Work out the finished part from the listing and answer in its coordinate system (mm). A direction names the side the tool comes from. Round coordinates to 2 decimals unless told otherwise and drop trailing zeros. Order: outer loops, then holes, each group sorted by start corner. A loop starts at its lowest first (then second) coordinate and runs counter-clockwise, first axis right, second up. Notation, with made-up numbers: M 40.5,46 L 92.5,46 A28 ccw 92.5,71 Z; hole C 69.5,66.25 d3. An arc over 180 degrees is marked long. Return JSON: item names as keys, results as strings.
from build123d import *

# Parameters (mm, degrees)
SKETCH1_R             = 14.29385
SKETCH1_R_2           = 11.1125
BOSS_EXTRUDE1_DEPTH   = 6.35
CROQUIS1_R            = 2.38125
CORTAR_EXTRUIR1_DEPTH = 50
CROQUIS2_R            = 5
CORTAR_EXTRUIR2_DEPTH = 3.175
CROQUIS4_R            = 5
CORTAR_EXTRUIR3_DEPTH = 3.175
CROQUIS5_R            = 2.38125
CORTAR_EXTRUIR5_DEPTH = 10
CROQUIS6_R            = 2.38125
CORTAR_EXTRUIR6_DEPTH = 10
CROQUIS7_R            = 5
CORTAR_EXTRUIR7_DEPTH = 3.17
CROQUIS8_R            = 17.5
CORTAR_EXTRUIR8_DEPTH = 10
CROQUIS9_R            = 2.5527
CORTAR_EXTRUIR9_DEPTH = 10


with BuildPart() as part:
    # Sketch1 → Boss-Extrude1 (new body)
    with BuildSketch(Plane.XY):
        with BuildLine():
            Line((0, 70), (310, 45))
            ThreePointArc((310, 45), (355, 0), (310, -45))
            Line((310, -45), (5.171398252, -69.808714643))
            ThreePointArc((5.171398252, -69.808714643), (-69.952162315, -2.587467389), (0, 70))
        make_face()
        Circle(SKETCH1_R, mode=Mode.SUBTRACT)
        with Locations((310, 0)):
            Circle(SKETCH1_R, mode=Mode.SUBTRACT)
        with Locations((162.878542763, 35)):
            Circle(SKETCH1_R_2, mode=Mode.SUBTRACT)
        with BuildLine():
            Line((107.898974887, 49.259511156), (143.314248041, 46.40344074))
            ThreePointArc((143.314248041, 46.40344074), (147.389908855, 43.644764005), (147.127454118, 38.730252238))
            Line((147.127454118, 38.730252238), (129.916226305, 11.754586611))
            ThreePointArc((129.916226305, 11.754586611), (125.651076231, 9.444205574), (121.433006579, 11.839462159))
            Line((121.433006579, 11.839462159), (103.228961238, 41.671198203))
            ThreePointArc((103.228961238, 41.671198203), (103.238833139, 46.896293531), (107.898974887, 49.259511156))
        make_face(mode=Mode.SUBTRACT)
        with BuildLine():
            Line((70.523244027, 6), (102.03004784, 6))
            ThreePointArc((102.03004784, 6), (106.3902351, 8.552804247), (106.298140539, 13.604493178))
            Line((106.298140539, 13.604493178), (96.590354482, 29.513051181))
            ThreePointArc((96.590354482, 29.513051181), (88.437172177, 34.296727565), (79.941746192, 30.151166228))
            Line((79.941746192, 30.151166228), (65.58297828, 10.229432452))
            ThreePointArc((65.58297828, 10.229432452), (67.271539685, 7.201787411), (70.523244027, 6))
        make_face(mode=Mode.SUBTRACT)
        with BuildLine():
            Line((219.623774494, 32.810522613), (206.130928429, 12.417497436))
            ThreePointArc((206.130928429, 12.417497436), (201.919524559, 10.176643248), (197.745901529, 12.48710226))
            Line((197.745901529, 12.48710226), (183.296864227, 35.133505128))
            ThreePointArc((183.296864227, 35.133505128), (183.227765467, 40.400743015), (187.913912204, 42.80669363))
            Line((187.913912204, 42.80669363), (215.855795571, 40.553315939))
            ThreePointArc((215.855795571, 40.553315939), (219.949772588, 37.757395035), (219.623774494, 32.810522613))
        make_face(mode=Mode.SUBTRACT)
        with BuildLine():
            Line((96.590354482, -29.513051181), (106.298140539, -13.604493178))
            ThreePointArc((106.298140539, -13.604493178), (106.3902351, -8.552804247), (102.03004784, -6))
            Line((102.03004784, -6), (70.523244027, -6))
            ThreePointArc((70.523244027, -6), (67.271539685, -7.201787411), (65.58297828, -10.229432452))
            Line((65.58297828, -10.229432452), (79.941746192, -30.151166228))
            ThreePointArc((79.941746192, -30.151166228), (88.437172177, -34.296727565), (96.590354482, -29.513051181))
        make_face(mode=Mode.SUBTRACT)
        with BuildLine():
            Line((187.913912204, -42.80669363), (215.855795571, -40.553315939))
            ThreePointArc((215.855795571, -40.553315939), (219.949772588, -37.757395035), (219.623774494, -32.810522613))
            Line((219.623774494, -32.810522613), (206.130928429, -12.417497436))
            ThreePointArc((206.130928429, -12.417497436), (201.919524559, -10.176643248), (197.745901529, -12.48710226))
            Line((197.745901529, -12.48710226), (183.296864227, -35.133505128))
            ThreePointArc((183.296864227, -35.133505128), (183.227765467, -40.400743015), (187.913912204, -42.80669363))
        make_face(mode=Mode.SUBTRACT)
        with BuildLine():
            Line((121.433006579, -11.839462159), (103.228961238, -41.671198203))
            ThreePointArc((103.228961238, -41.671198203), (103.238833139, -46.896293531), (107.898974887, -49.259511156))
            Line((107.898974887, -49.259511156), (143.314248041, -46.40344074))
            ThreePointArc((143.314248041, -46.40344074), (147.389908855, -43.644764005), (147.127454118, -38.730252238))
            Line((147.127454118, -38.730252238), (129.916226305, -11.754586611))
            ThreePointArc((129.916226305, -11.754586611), (125.651076231, -9.444205574), (121.433006579, -11.839462159))
        make_face(mode=Mode.SUBTRACT)
    extrude(amount=BOSS_EXTRUDE1_DEPTH)

    # Croquis1 → Cortar-Extruir1 (cut)
    with BuildSketch(Plane.XY.offset(6.35)):
        with Locations((98.995555235, -37.090103176)):
            Circle(CROQUIS1_R)
        with Locations((228.877351461, -26.519571404)):
            Circle(CROQUIS1_R)
    extrude(amount=-CORTAR_EXTRUIR1_DEPTH, mode=Mode.SUBTRACT)

    # Croquis2 → Cortar-Extruir2 (cut)
    with BuildSketch(Plane.XY.offset(6.35)):
        with Locations((98.995555235, -37.090103176)):
            Circle(CROQUIS2_R)
        with Locations((228.877351461, -26.519571404)):
            Circle(CROQUIS2_R)
    extrude(amount=-CORTAR_EXTRUIR2_DEPTH, mode=Mode.SUBTRACT)

    # Croquis4 → Cortar-Extruir3 (cut)
    with BuildSketch(Plane.XY.offset(6.35)):
        with Locations((162.878542763, -5)):
            Circle(CROQUIS4_R)
    extrude(amount=-CORTAR_EXTRUIR3_DEPTH, mode=Mode.SUBTRACT)

    # Croquis5 → Cortar-Extruir5 (cut)
    with BuildSketch(Plane.XY.offset(6.35)):
        with Locations((162.878542763, -5)):
            Circle(CROQUIS5_R)
    extrude(amount=-CORTAR_EXTRUIR5_DEPTH, mode=Mode.SUBTRACT)

    # Croquis6 → Cortar-Extruir6 (cut)
    with BuildSketch(Plane.XY.offset(6.35)):
        with Locations((65.84135797, 50.868973694)):
            Circle(CROQUIS6_R)
        with Locations((262.871569637, 39.210126075)):
            Circle(CROQUIS6_R)
    extrude(amount=-CORTAR_EXTRUIR6_DEPTH, mode=Mode.SUBTRACT)

    # Croquis7 → Cortar-Extruir7 (cut)
    with BuildSketch(Plane.XY.offset(6.35)):
        with Locations((65.84135797, 50.868973694)):
            Circle(CROQUIS7_R)
        with Locations((262.871569637, 39.210126075)):
            Circle(CROQUIS7_R)
    extrude(amount=-CORTAR_EXTRUIR7_DEPTH, mode=Mode.SUBTRACT)

    # Croquis8 → Cortar-Extruir8 (cut)
    with BuildSketch(Plane.XY.offset(6.35)):
        Circle(CROQUIS8_R)
    extrude(amount=-CORTAR_EXTRUIR8_DEPTH, mode=Mode.SUBTRACT)

    # Croquis9 → Cortar-Extruir9 (cut)
    with BuildSketch(Plane(origin=(0, 0, 0), x_dir=(-1, 0, 0), z_dir=(0, 0, -1))):
        with Locations((23.8125, 0)):
            Circle(CROQUIS9_R)
        with Locations((11.90625, -20.622229928)):
            Circle(CROQUIS9_R)
        with Locations((-11.90625, -20.622229928)):
            Circle(CROQUIS9_R)
        with Locations((-23.8125, 0)):
            Circle(CROQUIS9_R)
        with Locations((-11.90625, 20.622229928)):
            Circle(CROQUIS9_R)
        with Locations((11.90625, 20.622229928)):
            Circle(CROQUIS9_R)
    extrude(amount=-CORTAR_EXTRUIR9_DEPTH, mode=Mode.SUBTRACT)


solid = part.part
Item 1: Find section B-B (z = 4.75). State how many separate pieces and enclosed holes the cut face has, plus the area to 3 significant figures.
Output:
{"separate pieces": "1", "enclosed holes": "20", "area": "38,700 mm^2"}
Item 2: Find section C-C (x = 279.5). Determine the outline of the cut face in (y, z).
Output:
{"outline": "M -47.48,0 L 47.46,0 L 47.46,6.35 L -47.48,6.35 Z"}
Item 3: Which of the six approach directions +Z, -Z, +X, -X, +Y, -Y give full straight-line access (tool end or side, diameter ignored) to faces 5 (the flat face through (230, -29, 3.175)), 6 (the flat face through (159.72, -57.23, 3.13)), 7 (the flat face through (190.623, 23.652, 3.131))?
Output:
{"face 5": "+Z", "face 6": "+Z, -Z, +X, -Y", "face 7": "+Z, -Z"}
Item 4: The mould has two halves that part along X. Classify faces 1 (the flat face through (72.863, 20.33, 3.131)), 2 (the cylindrical face through (354.99, 0.99, 3.13)), 3 (the flat face through (145, 1, 0)), 4 (the flat face through (101.51, 21.45, 3.13)): pulls with the +X half, pulls with the -X half, needs draft (parallel to the pull), parting line crosses it, or undercut.
Output:
{"face 1": "undercut", "face 2": "pulls with the +X half", "face 3": "needs draft", "face 4": "undercut"}
Item 5: Find section A-A (x = -41.5). Determine the outline of the cut face in (y, z).
Output:
{"outline": "M -56.37,0 L 56.37,0 L 56.37,6.35 L -56.37,6.35 Z"}
Item 6: Each of these flat-tipped pins is pushed along its axis until it touches: pin 1 (5 mm diameter, centred on x = 164.5, y = -7.5, fed in from +Z); pin 2 (1.5 mm diameter, centred on y = -46.5, z = 5.5, fed in from -X); pin 3 (3 mm diameter, centred on x = 31.5, z = 1.5, fed in from -Y); pin 4 (1.5 mm diameter, centred on y = 40, z = 2.5, fed in from +X). Where does it stop, or does it pass through?
Output:
{"pin 1": "stops at z = 6.35", "pin 2": "stops at x = -52.98", "pin 3": "stops at y = -67.79", "pin 4": "stops at x = 332.01"}
Item 7: Consider line 1 along Y through (x, z) = (97.5, 1.5); line 2 along Y through (x, z) = (125.5, 4); line 3 along Y through (x, z) = (-11.5, 2.5). Determine where each line is inside the solid, lowest interval first. Write a range as [from, to].
Output:
{"line 1": "y = [-62.29, -38.94], [-35.24, -28.02], [-6, 6], [28.02, 62.14]", "line 2": "y = [-60.02, -47.84], [-9.45, 9.45], [47.84, 59.88]", "line 3": "y = [-69.05, -23.14], [-18.1, -13.19], [13.19, 18.1], [23.14, 69.05]"}
